from build123d import *

# Parameters (mm, degrees)
SKETCH_R             = 6.5
PAD_DEPTH            = 10
SKETCH001_W          = 8
SKETCH001_H          = 4.2
POCKET_DEPTH         = 10.001
SKETCH002_R          = 2.75
POCKET001_DEPTH      = 6.501
POCKET001_DEPTH_BACK = -6.501


with BuildPart() as part:
    # Sketch → Pad (new body)
    with BuildSketch(Plane.XY):
        Circle(SKETCH_R)
    extrude(amount=PAD_DEPTH)

    # Sketch001 (on Face3 of Pad) → Pocket (cut, through all)
    with BuildSketch(Plane.XY.offset(10)):
        Rectangle(SKETCH001_W, SKETCH001_H)
    extrude(amount=-POCKET_DEPTH, mode=Mode.SUBTRACT)

    # Sketch002 → Pocket001 (cut, two sides)
    with BuildSketch(Plane.XZ) as pocket001_sk:
        with Locations((0, 5)):
            Circle(SKETCH002_R)
    extrude(amount=-POCKET001_DEPTH, mode=Mode.SUBTRACT)
    extrude(pocket001_sk.sketch, amount=-POCKET001_DEPTH_BACK, mode=Mode.SUBTRACT)


solid = part.part
Source: CAD feature listing. Evaluate the final solid. Frame: model axes, mm. A direction names the side the tool comes from. Coordinates: 2 decimals unless noted, no trailing zeros. Order: outer loops, then holes, each group sorted by start corner. A loop starts at its lowest first (then second) coordinate and runs counter-clockwise, first axis right, second up. Notation, with made-up numbers: M 3.5,23.25 L 28.5,23.25 A5 cw 28.5,30.25 Z; hole C -8,85.25 d10. An arc over 180 degrees is marked long. Write each question's results on one line, items separated by ' | '. Start each with the question number.
1. Section A-A, the plane x = 0. Return the cut outline in (y, z), then the cut area to 3 significant figures.
2. Section B-B, the plane y = 0. Return the cut outline in (x, z), then the cut area to 3 significant figures.
3. Draft query along X for faces 3 (the face through (0, -3, 10)), 4 (the face through (6.2, 1.95, 4.93)), 5 (the face through (2.54, -4.27, 3.95)). Return one class per face: +X half, -X half, draft (parallel to the pull), parting line (faces both ways), or undercut.
4. Section D-D, the plane z = 5.5. Return the cut outline in (x, y).
5. Material intervals for L1, parallel to Z at x = 0, y = 3.8; L2, parallel to Z at x = 1.75, y = -4.75; L3, parallel to X at y = -4, z = 5, sorted ascending.
6. Reachability of faces 1 (the face through (-1.8, -2.1, 7.3)), 2 (the face through (0, -3, 0)) from +Z, -Z, +X, -X, +Y, -Y: full face, straight path, thin tool, end or side. Return the list, or none.
7. Pin query (flat end, axial travel): pin 1 (2 mm diameter, centred on x = 4, z = 6.5, fed in from -Y); pin 2 (1 mm diameter, centred on x = -1.5, z = 8.5, fed in from +Y); pin 3 (6 mm diameter, centred on y = 5, z = 8.5, fed in from +X); pin 4 (1.5 mm diameter, centred on x = -0.5, y = -2, fed in from +Z). Return the tip coordinate at first contact, or that it passes through.
8. Section C-C, the plane z = 9. Return the cut outline in (x, y).
Solution:
1) outline: M -6.5,0 L -2.1,0 L -2.1,2.25 L -6.5,2.25 Z; M -6.5,7.75 L -2.1,7.75 L -2.1,10 L -6.5,10 Z; M 2.1,0 L 6.5,0 L 6.5,2.25 L 2.1,2.25 Z; M 2.1,7.75 L 6.5,7.75 L 6.5,10 L 2.1,10 Z | area: 39.6 mm²
2) outline: M -6.5,0 L -4,0 L -4,10 L -6.5,10 Z; M 4,0 L 6.5,0 L 6.5,10 L 4,10 Z | area: 50.0 mm²
3) face 3: draft | face 4: parting line | face 5: undercut
4) outline: M -4,-2.1 L -4,2.1 L -2.7,2.1 L -2.7,5.91 A6.5 ccw -2.7,-5.91 L -2.7,-2.1 Z; M 2.7,-5.91 A6.5 ccw 2.7,5.91 L 2.7,2.1 L 4,2.1 L 4,-2.1 L 2.7,-2.1 Z
5) L1: 0 to 2.25, 7.75 to 10 | L2: 0 to 2.88, 7.12 to 10 | L3: -5.12 to -2.75, 2.75 to 5.12
6) face 1: +Z, -Z | face 2: -Z, +X, -X, +Y, -Y
7) pin 1: y = -5.77 | pin 2: y = 6.42 | pin 3: x = 6.18 | pin 4: z = 10
8) outline: C 0,0 d13; hole M -4,-2.1 L 4,-2.1 L 4,2.1 L -4,2.1 Z
